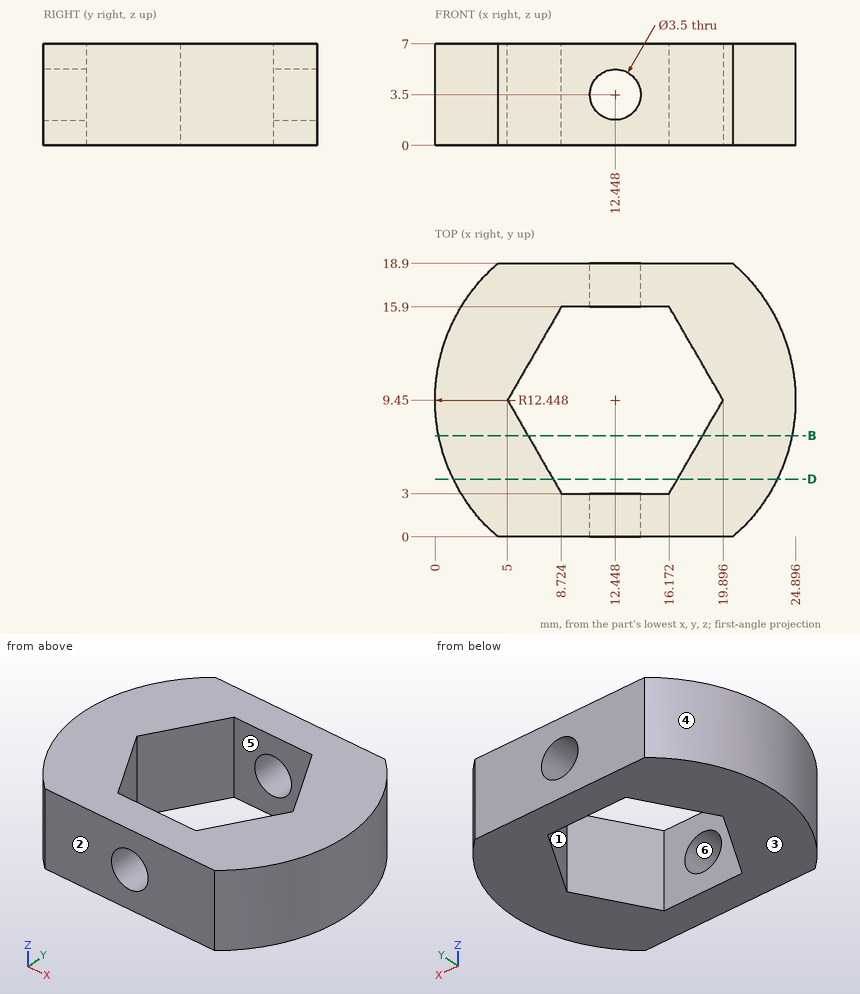
Study the drawing (mm; zero at the part's minimum x, y, z) and answer. A direction names the side the tool comes from. Round coordinates to 2 decimals unless told otherwise and drop trailing zeros. Write each loop counter-clockwise with the first axis right and the second up, starting at its lowest first coordinate (ties: lowest second). Pieces come first, ordered by that corner, then holes.
1) Which of the six approach directions +Z, -Z, +X, -X, +Y, -Y give full straight-line access (tool end or side, diameter ignored) to the marked faces 1 and 2?
2) A cutting plane is placed at B-B on y = 7. Determine the outline of the cut face in (x, z) (1 decimal), and give its area (3 significant figures).
3) A cutting plane is placed at D-D on y = 4. Determine the outline of the cut face in (x, z).
4) Consider probe 1 along Y at (x, z) = (9.5, 2.75); probe 2 along Z at (x, y) = (14, 17.25) (1 decimal); probe 3 along X at (y, z) = (16.5, 3) (1 decimal). Determine where each line is inside the solid, lowest interval first.
5) Determine the mould class of the marked faces 3, 4, 5 and 6 for opening direction X: pulls with the +X half, pulls with the -X half, needs draft (parallel to the pull), parting line crosses it, or undercut.
Entries:
1. face 1: +Z, -Z
1. face 2: +Z, -Z, +X, -X, -Y
2. outline: (0.2, 0) - (6.4, 0) - (6.4, 7) - (0.2, 7) - close; (18.5, 0) - (24.7, 0) - (24.7, 7) - (18.5, 7) - close
2. area: 86.4 mm2
3. outline: (1.26, 0) - (8.15, 0) - (8.15, 7) - (1.26, 7) - close; (16.75, 0) - (23.64, 0) - (23.64, 7) - (16.75, 7) - close
4. probe 1: y = 0 to 3, 15.9 to 18.9
4. probe 2: z = 0 to 2.7, 4.3 to 7
4. probe 3: x = 2.2 to 10.8, 14.1 to 22.7
5. face 3: needs draft
5. face 4: pulls with the -X half
5. face 5: undercut
5. face 6: undercut
